Could you check a few things on this model? Use its own coordinates, in mm. A direction names the side the tool comes from. Give positions to 0.01 mm unless a question says otherwise; leave off trailing zeros. Order: outer loops, then holes, each group sorted by start corner. A loop starts at its lowest first (then second) coordinate and runs counter-clockwise, first axis right, second up. Notation, with made-up numbers: (-26.75, 49) - (13.25, 49) arc R9 ccw to (13.25, 60) - close; hole circle Ø8 at (73.5, -5). An arc over 180 degrees is marked (long way). Put each result on its own line as item: value.
from build123d import *

# Parameters (mm, degrees)
SKETCH1_W           = 22
SKETCH1_H           = 55
SKETCH1_R           = 5.25
SKETCH1_W_2         = 4
SKETCH1_H_2         = 2.5
BOSS_EXTRUDE1_DEPTH = 18
SKETCH2_R           = 5.25
CUT_EXTRUDE1_DEPTH  = 62.911226769
SKETCH3_R           = 4
CUT_EXTRUDE2_DEPTH  = 20
SKETCH4_R           = 11
CUT_EXTRUDE3_DEPTH  = 2
FILLET3_R           = 2
FILLET2_R           = 2
FILLET4_R           = 2


# Some blends are built 0.0001 mm under size
with BuildPart() as part:
    # Sketch1 → Boss-Extrude1 (new body)
    with BuildSketch(Plane.XY):
        with Locations((11, 27.5)):
            Rectangle(SKETCH1_W, SKETCH1_H)
        with Locations((11, 12)):
            Circle(SKETCH1_R, mode=Mode.SUBTRACT)
        with Locations((11, 34)):
            Circle(SKETCH1_R, mode=Mode.SUBTRACT)
        with Locations((11, 45)):
            Rectangle(SKETCH1_W_2, SKETCH1_H_2, mode=Mode.SUBTRACT)
    extrude(amount=-BOSS_EXTRUDE1_DEPTH)

    # Sketch2 → Cut-Extrude1 (cut, through all)
    with BuildSketch(Plane.ZY):
        with Locations((-9, 23)):
            Circle(SKETCH2_R)
    extrude(amount=-CUT_EXTRUDE1_DEPTH, mode=Mode.SUBTRACT)

    # Sketch3 → Cut-Extrude2 (cut)
    with BuildSketch(Plane(origin=(0, 0, 0), x_dir=(0, 0, -1), z_dir=(1, 0, 0))):
        with Locations((9, 53.5)):
            Circle(SKETCH3_R)
    extrude(amount=CUT_EXTRUDE2_DEPTH, mode=Mode.SUBTRACT)

    # Sketch4 → Cut-Extrude3 (cut)
    with BuildSketch(Plane(origin=(22, 0, 0), x_dir=(0, 0, -1), z_dir=(1, 0, 0))):
        with Locations((9, 23)):
            Circle(SKETCH4_R)
    extrude(amount=-CUT_EXTRUDE3_DEPTH, mode=Mode.SUBTRACT)

    # Fillet3
    fillet3_edges = [part.edges().sort_by_distance(p)[0] for p in [
        (22, 12, -9),
        (22, 34, -9),
        (22, 8.33772234, -18),
        (22, 8.33772234, 0),
        (22, 42.16227766, -18),
        (22, 42.16227766, 0),
        (11, 55, -18),
        (11, 55, 0),
    ]]
    fillet(fillet3_edges, radius=FILLET3_R - 0.0001)  # a hair under: the kernel refuses the full size

    # Fillet2
    fillet2_edges = [part.edges().sort_by_distance(p)[0] for p in [
        (11, 46.25, -18),
        (11, 46.25, 0),
    ]]
    fillet(fillet2_edges, radius=FILLET2_R)

    # Fillet4
    # the kernel refuses this fillet: 2 mm, written as the material it takes off along each edge
    with BuildSketch(Plane(origin=(20, 53, -18), x_dir=(0, 1, 0), z_dir=(-1, 0, 0))) as fillet4_piece_1:
        with BuildLine():
            CenterArc((0.0001, -1.9999), 1.9999, 0, 90)
            Line((2, -1.9999), (2, 0))
            Line((2, 0), (0.0001, 0))
        make_face()
    revolve(axis=Axis((20, 53, -18), (0, 0, -1)), revolution_arc=90, mode=Mode.SUBTRACT)
    with BuildSketch(Plane(origin=(20, 53, 0), x_dir=(1, 0, 0), z_dir=(0, -1, 0))) as fillet4_piece_2:
        with BuildLine():
            CenterArc((0.0001, -1.9999), 1.9999, 0, 90)
            Line((2, -1.9999), (2, 0))
            Line((2, 0), (0.0001, 0))
        make_face()
    revolve(axis=Axis((20, 53, 0), (0, 0, 1)), revolution_arc=90, mode=Mode.SUBTRACT)
    with BuildSketch(Plane(origin=(22, 55, 0), x_dir=(0, -1, 0), z_dir=(0, 0, -1))) as fillet4_piece_3:
        with BuildLine():
            CenterArc((FILLET4_R, FILLET4_R), FILLET4_R, 180, 90)
            Line((0, FILLET4_R), (0, 0))
            Line((0, 0), (FILLET4_R, 0))
        make_face()
    extrude(amount=18, mode=Mode.SUBTRACT)


solid = part.part
1) We'd pull the mould along Z, two halves only. Please class faces 4 (the cylindrical face through (9.86, 18.34, -6.58)), 5 (the flat face through (11, 43.75, -9)), 6 (the cylindrical face through (21.4, 41.33, -17.43)): pulls with the +Z half, pulls with the -Z half, needs draft (parallel to the pull), parting line crosses it, or undercut.
Filled in:
face 4: undercut
face 5: needs draft
face 6: pulls with the -Z half
2) Suppose I cut it at C-C, the plane y = 23. List the corners of the cut face in (x, z) for me, and give its area (3 significant figures).
Filled in:
outline: (0, -18) - (20, -18) - (20, -14.25) - (0, -14.25) - close; (0, -3.75) - (20, -3.75) - (20, 0) - (0, 0) - close
area: 150 mm^2
3) I'm going to push a flat-ended pin straight in: pin 1 (3 mm diameter, centred on y = 53.5, z = -8, fed in from -X). Where does the tip first touch, or does it pass through?
Filled in:
pin 1: stops at x = 20
4) If I drill on line 1 (Y direction, x = 11, z = -8.5); line 2 (Y direction, x = 11, z = -10.5); line 3 (Y direction, x = 13.75, z = -9), over which ranges is the centre line in solid material (lowest first)? Write a range as [from, to].
Filled in:
line 1: y = [0, 6.75], [17.25, 17.77], [28.23, 28.75], [39.25, 43.75], [46.25, 49.53]
line 2: y = [0, 6.75], [17.25, 17.97], [28.03, 28.75], [39.25, 43.75], [46.25, 49.79]
line 3: y = [0, 7.53], [16.47, 17.75], [28.25, 29.53], [38.47, 49.5]
5) Suppose I cut it at B-B, the plane x = 11. List the corners of the cut face in (y, z) for me.
Filled in:
outline: (0, -18) - (6.75, -18) - (6.75, 0) - (0, 0) - close; (17.25, -18) - (28.75, -18) - (28.75, 0) - (17.25, 0) - close; (39.25, -18) - (43.75, -18) - (43.75, 0) - (39.25, 0) - close; (46.25, -16) arc R2 ccw to (48.25, -18) - (53, -18) arc R2 ccw to (55, -16) - (55, -12.71) arc R4 cw (long way) to (55, -5.29) - (55, -2) arc R2 ccw to (53, 0) - (48.25, 0) arc R2 ccw to (46.25, -2) - close; hole circle Ø10.5 at (23, -9)
6) Suppose I cut it at D-D, the plane x = 4.5. List the corners of the cut face in (y, z) for me.
Filled in:
outline: (0, -18) - (53, -18) arc R2 ccw to (55, -16) - (55, -12.71) arc R4 cw (long way) to (55, -5.29) - (55, -2) arc R2 ccw to (53, 0) - (0, 0) - close; hole circle Ø10.5 at (23, -9)
7) Which directions (+Z, -Z, +X, -X, +Y, -Y) give clear straight access to the entire face, cutting with the end or side of a thin tool? Please do faces 1 (the cylindrical face through (9.9, 49.5, -8.9)), 2 (the flat face through (10, 27, -18)), 3 (the flat face through (20, 28, -6.9)).
Filled in:
face 1: -X
face 2: -Z, +X, -X, +Y, -Y
face 3: +X
8) Suppose I cut it at A-A, the plane z = -9. State how many separate pieces and enclosed holes the cut face has, and give its area (3 significant figures).
Filled in:
separate pieces: 2
enclosed holes: 3
area: 660 mm^2
